Job drawing, mm, ordinate dimensions from the low corner. One solid piece. A direction names the side the tool comes from. Give positions to 0.01 mm unless a question says otherwise; leave off trailing zeros. Write each loop counter-clockwise with the first axis right and the second up, starting at its lowest first coordinate (ties: lowest second). Pieces come first, ordered by that corner, then holes. Notation, with made-up numbers: (-17.5, 63) - (6.5, 63) arc R22 ccw to (6.5, 92) - close; hole circle Ø1 at (46.25, 66.5). An arc over 180 degrees is marked (long way). Use a Markdown table: item, result. Add a question column.
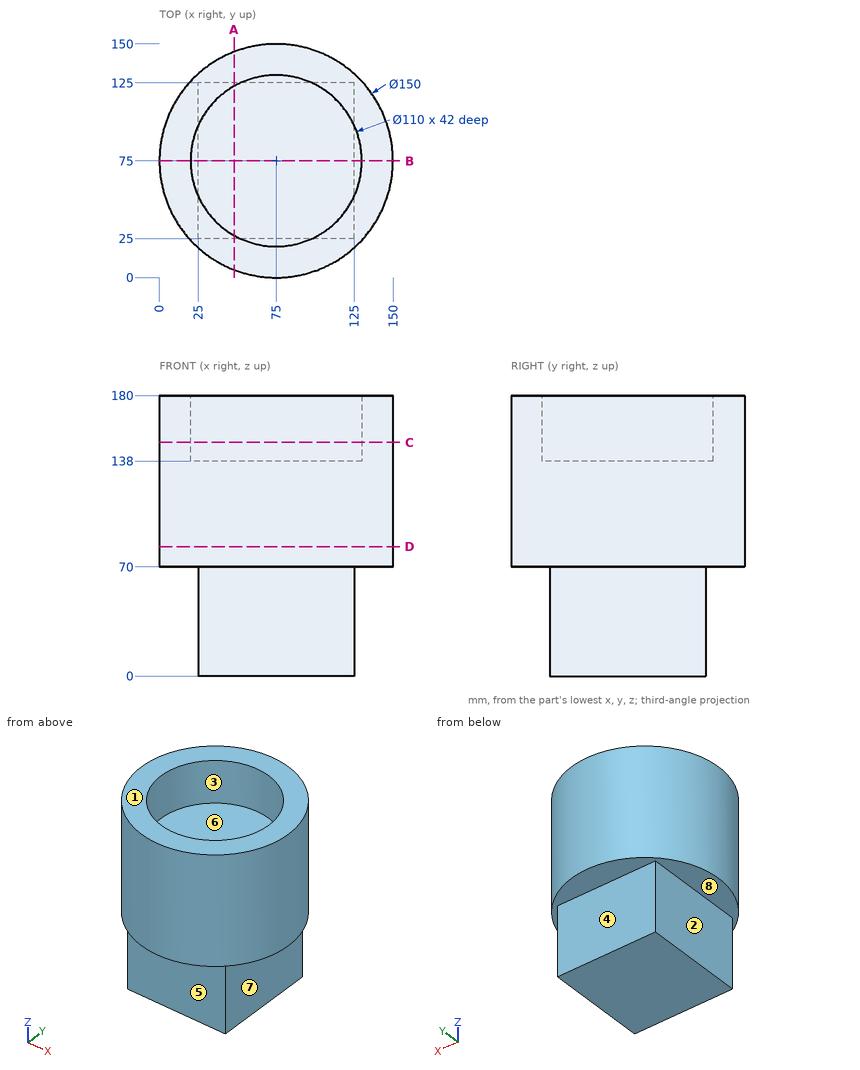
(1) Two-plate mould, pull along X, no slides. Class the marked faces 6, 7 and 8: +X half, -X half, draft (parallel to the pull), parting line (faces both ways), or undercut.
(2) Band-saw the part on D-D (z = 83). Write the cut outline in (x, y), then the cut area to 3 significant figures.
(3) Which spindle directions (+Z, -Z, +X, -X, +Y, -Y) get a long thin tool onto all of the face, cutting with end or side? Do the marked faces 1, 2, 3, 4 and 5. Say none if no direction does.
(4) Probe probe 1 along Y at (x, z) = (75, 163); probe 2 along X at (y, z) = (76, 157); probe 3 along Y at (x, z) = (66.5, 65). List the from-to ranges inside material, lowest first. Write a range as [from, to].
(5) Band-saw the part on C-C (z = 150). Write the cut outline in (x, y).
(6) Band-saw the part on B-B (y = 75). Write the cut outline in (x, z), then the cut area to 3 significant figures.
(7) Band-saw the part on A-A (x = 48). Write the cut outline in (y, z).
(8) Flat gauge pins, fed straight in: pin 1 (2 mm diameter, centred on x = 115, z = 155.5, fed in from +Y); pin 2 (6 mm diameter, centred on x = 41, y = 115.5, fed in from +Z); pin 3 (1.5 mm diameter, centred on y = 63, z = 149.5, fed in from -X); pin 4 (1.5 mm diameter, centred on x = 58, z = 112, fed in from +Y). Where does each tip first touch, or does it go through?
Model answer:
| question | item | result |
|---|---|---|
| 1 | face 6 | undercut |
| 1 | face 7 | +X half |
| 1 | face 8 | draft |
| 2 | outline | circle Ø150 at (75, 75) |
| 2 | area | 17,700 mm^2 |
| 3 | face 1 | +Z, +X, -X, +Y, -Y |
| 3 | face 2 | -Z, -X, +Y, -Y |
| 3 | face 3 | +Z |
| 3 | face 4 | -Z, +X, -X, +Y |
| 3 | face 5 | -Z, +X, -X, -Y |
| 4 | probe 1 | y = [0, 20], [130, 150] |
| 4 | probe 2 | x = [0.01, 20.01], [129.99, 149.99] |
| 4 | probe 3 | y = [25, 125] |
| 5 | outline | circle Ø150 at (75, 75); hole circle Ø110 at (75, 75) |
| 6 | outline | (0, 70) - (25, 70) - (25, 0) - (125, 0) - (125, 70) - (150, 70) - (150, 180) - (130, 180) - (130, 138) - (20, 138) - (20, 180) - (0, 180) - close |
| 6 | area | 18,900 mm^2 |
| 7 | outline | (5.03, 70) - (25, 70) - (25, 0) - (125, 0) - (125, 70) - (144.97, 70) - (144.97, 180) - (122.92, 180) - (122.92, 138) - (27.08, 138) - (27.08, 180) - (5.03, 180) - close |
| 8 | pin 1 | stops at y = 139.06 |
| 8 | pin 2 | stops at z = 180 |
| 8 | pin 3 | stops at x = 0.85 |
| 8 | pin 4 | stops at y = 148.22 |
